Part model, mm, in its own coordinate system. Round coordinates to 2 decimals unless told otherwise and drop trailing zeros. Write each loop counter-clockwise with the first axis right and the second up, starting at its lowest first coordinate (ties: lowest second). Pieces come first, ordered by that corner, then holes.
Autodesk Inventor part; units mm, degrees
ref_plane "YZ Plane" through (0, 0, 0) normal (1, 0, 0) x (0, 1, 0)
ref_plane "XZ Plane" through (0, 0, 0) normal (0, 1, 0) x (-1, 0, 0)
ref_plane "XY Plane" through (0, 0, 0) normal (0, 0, 1) x (1, 0, 0)
sketch "Sketch1" plane through (0, 0, 0) normal (0, 0, 1) x (1, 0, 0)
  line L0 (9.525, 0) -> (9.525, 19.05)
  line L1 (0, 19.05) -> (0, 0)
  arc A0 (9.525, 19.05) -> (0, 19.05) centre (4.7625, 19.05) ccw
  arc A1 (0, 0) -> (9.525, 0) centre (4.7625, 0) ccw
  dimension "d0" = 9.525
  dimension "d1" = 19.05
extrude "Extrusion1" add sketch "Sketch1" along normal blind 2.54
sketch "Sketch2" plane through (0, 0, 2.54) normal (0, 0, 1) x (1, 0, 0)
  arc A0 (9.525, 19.05) -> (0, 19.05) centre (4.7625, 19.05) ccw
  point P0 (0, 0)
  dimension "d18" = 4.7625
hole "Hole1" at (4.7625, 19.05, 2.54) direction (0, 0, -1) diameter 2.9 end through all
sketch "Sketch3" plane through (0, 0, 2.54) normal (0, 0, 1) x (1, 0, 0)
  circle A0 centre (4.7625, 19.05) radius 1.45
  point P0 (0, 0)
  point P1 (4.7752, 0)
  dimension "d19" = 4.7752
  dimension "d20" = 19.05
  dimension "d21" = 2.9
hole "Hole2" at (4.7752, 0, 2.54) direction (0, 0, -1) diameter 3.9 end through all
Q1. Drop a flat-ended pin along its axis: pin 1 (2.5 mm diameter, centred on x = 4.76, y = 19.05, fed in from +Z). Give the stop position or say it passes through.
Values follow:
pin 1: passes through
Q2. Mould opens along X. For faces 1 (the flat face through (9.525, 9, 1)), 2 (the cylindrical face through (4.66, 23.81, 1.25)), 3 (the cylindrical face through (3.46, 1.44, 1.25)), 4 (the cylindrical face through (3.783, 20.119, 1.252)) say: +X half, -X half, draft (parallel to the pull), parting line (faces both ways), or undercut.
Values follow:
face 1: +X half
face 2: parting line
face 3: undercut
face 4: undercut
Q3. Cut at D-D on y = 22. Write the cut outline in (x, z), plus the area to 3 significant figures.
Values follow:
outline: (1.02, 0) - (8.5, 0) - (8.5, 2.54) - (1.02, 2.54) - close
area: 19.0 mm2
Q4. Cut at A-A on y = 1.25. Write the cut outline in (x, z) (3 decimals), plus the area to 3 significant figures.
Values follow:
outline: (0, 0) - (3.279, 0) - (3.279, 2.54) - (0, 2.54) - close; (6.272, 0) - (9.525, 0) - (9.525, 2.54) - (6.272, 2.54) - close
area: 16.6 mm2
Q5. Cut at B-B on x = 5.25. Write the cut outline in (y, z).
Values follow:
outline: (-4.74, 0) - (-1.89, 0) - (-1.89, 2.54) - (-4.74, 2.54) - close; (1.89, 0) - (17.68, 0) - (17.68, 2.54) - (1.89, 2.54) - close; (20.42, 0) - (23.79, 0) - (23.79, 2.54) - (20.42, 2.54) - close
Q6. Wall check: L1, parallel to Y at x = 3.75, z = 0.8; L2, parallel to Y at x = 6, z = 0.85; L3, parallel to X at y = 0, z = 1.9 (3 decimals). Give the ranges that are in metal, low to high.
Values follow:
L1: y = -4.65 to -1.66, 1.66 to 18.01, 20.09 to 23.7
L2: y = -4.6 to -1.52, 1.52 to 18.29, 19.81 to 23.65
L3: x = 0 to 2.825, 6.725 to 9.525
Q7. Cut at C-C on z = 1.35. State how many separate pieces and enclosed holes the cut face has, plus the area to 3 significant figures.
Values follow:
separate pieces: 1
enclosed holes: 2
area: 234 mm2
